Drawing for the job (mm, zero at the part's lowest x, y, z). A direction names the side the tool comes from. Coordinates: 2 decimals unless noted, no trailing zeros. Order: outer loops, then holes, each group sorted by start corner. A loop starts at its lowest first (then second) coordinate and runs counter-clockwise, first axis right, second up.
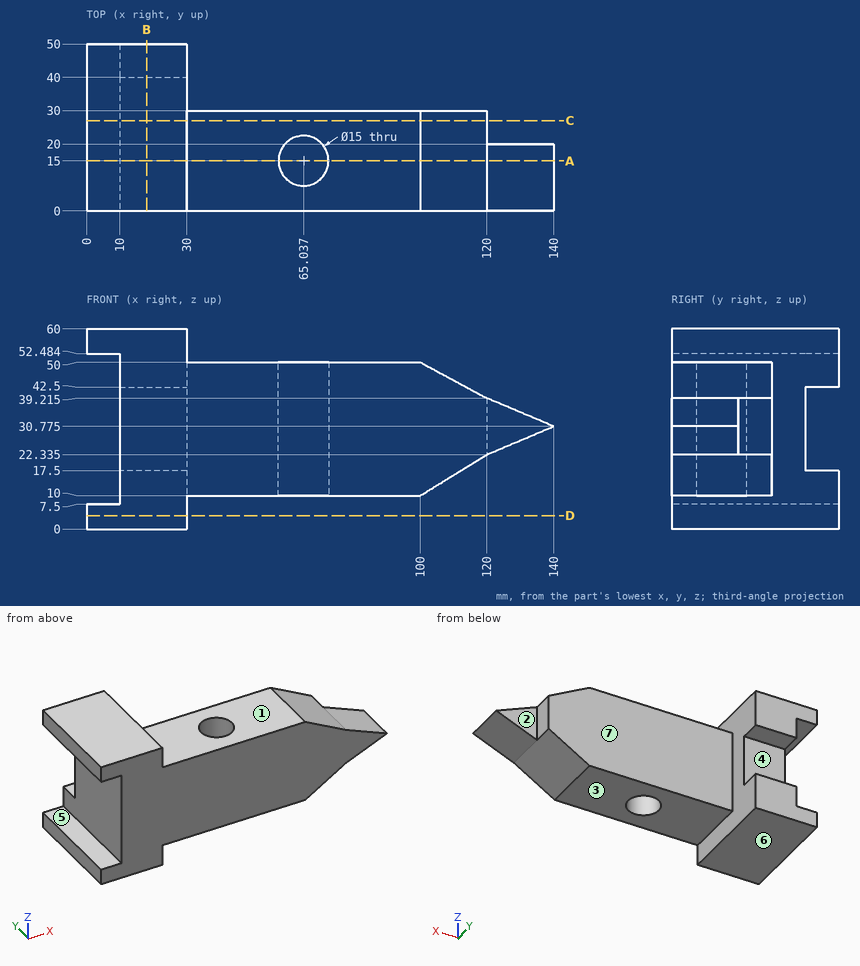
1) Slice it at A-A (y = 15). List the corners of the cut face in (x, z) (1 decimal).
2) Slice it at D-D (z = 4). List the corners of the cut face in (x, y), plus the area to 3 significant figures.
3) Drill centre lines: probe 1 along Y at (x, z) = (88, 45.5); probe 2 along X at (y, z) = (48.5, 51); probe 3 along X at (y, z) = (24, 37). Where is each one in solid material? Low to high.
4) Pin check, flat tips, straight feed: P1, Ø5, axis at y = 43, z = 22, coming from the +X side; P2, Ø24, axis at x = 65.04, y = 15, coming from the -Z side; P3, Ø13.5, axis at y = 20.5, z = 38, coming from the -X side; P4, Ø2, axis at x = 86.5, z = 22.5, coming from the +Y side. Stop position of each tip, or through.
5) Which spindle directions (+Z, -Z, +X, -X, +Y, -Y) get a long thin tool onto all of the face, cutting with end or side? Do the marked faces 1, 2, 3 and 4. Say none if no direction does.
6) Slice it at B-B (x = 18). List the corners of the cut face in (y, z).
7) Slice it at C-C (y = 27). List the corners of the cut face in (x, z) (1 decimal).
8) Two-plate mould, pull along Z, no slides. Class the marked faces 5, 6 and 7: released by +Z, released by -Z, zero draft, split by the parting line, or undercut.
Worked out:
1. outline: (0, 0) - (30, 0) - (30, 10) - (57.5, 10) - (57.5, 50) - (30, 50) - (30, 60) - (0, 60) - (0, 52.5) - (10, 52.5) - (10, 7.5) - (0, 7.5) - close; (72.5, 10) - (100, 10) - (120, 22.3) - (140, 30.8) - (120, 39.2) - (100, 50) - (72.5, 50) - close
2. outline: (0, 0) - (30, 0) - (30, 50) - (0, 50) - close
2. area: 1,500 mm2
3. probe 1: y = 0 to 30
3. probe 2: x = 10 to 30
3. probe 3: x = 10 to 120
4. P1: passes through
4. P2: stops at z = 10
4. P3: stops at x = 10
4. P4: stops at y = 30
5. face 1: +Z, +X, +Y, -Y
5. face 2: +Z, -Z, +X, +Y
5. face 3: -Z, +X, +Y, -Y
5. face 4: +X, -X, +Y
6. outline: (0, 0) - (50, 0) - (50, 17.5) - (40, 17.5) - (40, 42.5) - (50, 42.5) - (50, 60) - (0, 60) - close
7. outline: (0, 0) - (30, 0) - (30, 10) - (100, 10) - (120, 22.3) - (120, 39.2) - (100, 50) - (30, 50) - (30, 60) - (0, 60) - (0, 52.5) - (10, 52.5) - (10, 7.5) - (0, 7.5) - close
8. face 5: undercut
8. face 6: released by -Z
8. face 7: zero draft
